Could you check a few things on this model? Use its own coordinates, in mm. A direction names the side the tool comes from. Round coordinates to 2 decimals unless told otherwise and drop trailing zeros. Loops run counter-clockwise (first coordinate to the right, second up) from the corner with the lowest first, then second, coordinate; pieces in that order, holes last.
from build123d import *

# Parameters (mm, degrees)
SKETCH1_R           = 18.875
SKETCH1_R_2         = 15.875
BOSS_EXTRUDE1_DEPTH = 47.85
SKETCH2_R           = 38
BOSS_EXTRUDE2_DEPTH = 30
SKETCH3_R           = 15.875
CUT_EXTRUDE1_DEPTH  = 47.85
SKETCH4_W           = 76
SKETCH4_H           = 20
CUT_EXTRUDE2_DEPTH  = 47.85
SKETCH5_R           = 2.65
CUT_EXTRUDE3_DEPTH  = 47.85
SKETCH11_R          = 1
CUT_EXTRUDE4_DEPTH  = 30
SKETCH12_R          = 4.7625
CUT_EXTRUDE5_DEPTH  = 8
SKETCH13_W          = 2.1
SKETCH13_H          = 3.2
SKETCH13_W_2        = 4.5
SKETCH13_H_2        = 2.2
SKETCH18_R          = 3.125
CUT_EXTRUDE8_DEPTH  = 30
SKETCH19_R          = 5.25
CUT_EXTRUDE9_DEPTH  = 27
SKETCH27_R          = 6.225
CUT_EXTRUDE12_DEPTH = 1.6
CHAMFER1_SIZE       = 2
SKETCH28_W          = 76
SKETCH28_H          = 20
CUT_EXTRUDE13_DEPTH = 1


with BuildPart() as part:
    # Sketch1 → Boss-Extrude1 (new body)
    with BuildSketch(Plane.XY):
        Circle(SKETCH1_R)
        Circle(SKETCH1_R_2, mode=Mode.SUBTRACT)
    extrude(amount=BOSS_EXTRUDE1_DEPTH)

    # Sketch2 → Boss-Extrude2 (add)
    with BuildSketch(Plane.XY.offset(47.85)):
        Circle(SKETCH2_R)
    extrude(amount=BOSS_EXTRUDE2_DEPTH)

    # Sketch3 → Cut-Extrude1 (cut)
    with BuildSketch(Plane(origin=(0, 0, 47.85), x_dir=(-1, 0, 0), z_dir=(0, 0, -1))):
        with Locations(Location((0, 0, 0), (0, 0, 180))):
            Circle(SKETCH3_R)
    extrude(amount=-CUT_EXTRUDE1_DEPTH, mode=Mode.SUBTRACT)

    # Sketch4 → Cut-Extrude2 (cut)
    with BuildSketch(Plane(origin=(0, 0, 0), x_dir=(1, 0, 0), z_dir=(0, 1, 0))):
        with Locations((0, -67.85)):
            Rectangle(SKETCH4_W, SKETCH4_H)
    extrude(amount=-CUT_EXTRUDE2_DEPTH, mode=Mode.SUBTRACT)

    # Sketch5 → Cut-Extrude3 (cut)
    with BuildSketch(Plane(origin=(0, 0, 0), x_dir=(-1, 0, 0), z_dir=(0, -1, 0))):
        with Locations(Location((26.9375, -67.85, 0), (0, 0, 90))):
            Circle(SKETCH5_R)
        with Locations(Location((-26.9375, -67.85, 0), (0, 0, 90))):
            Circle(SKETCH5_R)
    extrude(amount=-CUT_EXTRUDE3_DEPTH, mode=Mode.SUBTRACT)

    # Sketch11 → Cut-Extrude4 (cut)
    with BuildSketch(Plane.XY.offset(77.85)):
        with Locations((0, 28.5)):
            Circle(SKETCH11_R)
    extrude(amount=-CUT_EXTRUDE4_DEPTH, mode=Mode.SUBTRACT)

    # Sketch12 → Cut-Extrude5 (cut)
    with BuildSketch(Plane.XY.offset(77.85)):
        with Locations((0, 28.5)):
            Circle(SKETCH12_R)
    extrude(amount=-CUT_EXTRUDE5_DEPTH, mode=Mode.SUBTRACT)

    # Sketch13 → Cut-Revolve1 (revolve, cut)
    with BuildSketch(Plane(origin=(0, 0, 0), x_dir=(0, 0, -1), z_dir=(1, 0, 0)), mode=Mode.PRIVATE) as cut_revolve1_sk:
        with Locations((-14.85, 18.875)):
            Rectangle(SKETCH13_W, SKETCH13_H)
        with Locations((-22.85, 18.875)):
            Rectangle(SKETCH13_W, SKETCH13_H)
        with Locations((-35.85, 18.875)):
            Rectangle(SKETCH13_W, SKETCH13_H)
        with Locations((-39.85, 18.875)):
            Rectangle(SKETCH13_W, SKETCH13_H)
        with Locations((-29.85, 18.375)):
            Rectangle(SKETCH13_W_2, SKETCH13_H_2)
    revolve(cut_revolve1_sk.sketch.rotate(Axis((0, 0, 0), (0, 0, 1)), 90), axis=Axis((0, 0, 0), (0, 0, 1)), mode=Mode.SUBTRACT)

    # Sketch18 → Cut-Extrude8 (cut)
    with BuildSketch(Plane.XY.offset(77.85)):
        with Locations((27.105110714, 8.80698434)):
            Circle(SKETCH18_R)
        with Locations((16.75187969, -23.05698434)):
            Circle(SKETCH18_R)
        with Locations((-16.75187969, -23.05698434)):
            Circle(SKETCH18_R)
        with Locations((-27.105110714, 8.80698434)):
            Circle(SKETCH18_R)
    extrude(amount=-CUT_EXTRUDE8_DEPTH, mode=Mode.SUBTRACT)

    # Sketch19 → Cut-Extrude9 (cut)
    with BuildSketch(Plane.XY.offset(77.85)):
        with Locations((27.105110714, 8.80698434)):
            Circle(SKETCH19_R)
        with Locations((16.75187969, -23.05698434)):
            Circle(SKETCH19_R)
        with Locations((-16.75187969, -23.05698434)):
            Circle(SKETCH19_R)
        with Locations((-27.105110714, 8.80698434)):
            Circle(SKETCH19_R)
    extrude(amount=-CUT_EXTRUDE9_DEPTH, mode=Mode.SUBTRACT)

    # Sketch27 → Cut-Extrude12 (cut)
    with BuildSketch(Plane(origin=(0, 0, 47.85), x_dir=(-1, 0, 0), z_dir=(0, 0, -1))):
        with Locations((0, 28.5)):
            Circle(SKETCH27_R)
    extrude(amount=-CUT_EXTRUDE12_DEPTH, mode=Mode.SUBTRACT)

    # Chamfer1
    chamfer1_edges = [part.edges().sort_by_distance(p)[0] for p in [
        (0, 38, 77.85),
    ]]
    chamfer(chamfer1_edges, length=CHAMFER1_SIZE)

    # Sketch28 → Cut-Extrude13 (cut)
    with BuildSketch(Plane(origin=(0, 0, 0), x_dir=(-1, 0, 0), z_dir=(0, -1, 0))):
        with Locations((0, -67.85)):
            Rectangle(SKETCH28_W, SKETCH28_H)
    extrude(amount=-CUT_EXTRUDE13_DEPTH, mode=Mode.SUBTRACT)


solid = part.part
Item 1: For faces 1 (the flat face through (-17.4, -7.9, 47.85)), 2 (the flat face through (-29, 1, 65)), 3 (the flat face through (17, 6, 13.8)), 4 (the cylindrical face through (-0.13, 29.49, 59.79)), which set-ups out of +Z, -Z, +X, -X, +Y, -Y let a thin tool reach every point of the face, with its end or its side?
Results list:
face 1: -Z
face 2: +Z, +X, -X, -Y
face 3: none
face 4: +Z, -Z
Item 2: We'd pull the mould along Y, two halves only. Please class faces 5 (the cylindrical face through (-29.59, 6.91, 49.37)), 6 (the cylindrical face through (12.88, -19.51, 54.4)), 7 (the cylindrical face through (18.003, 5.67, 18.809)), 8 (the flat face through (17, 6, 36.9)): released by +Y, released by -Y, zero draft, split by the parting line, or undercut.
Results list:
face 5: undercut
face 6: undercut
face 7: split by the parting line
face 8: zero draft
Item 3: If we section it at C-C, the plane z = 54.5: Please give me the cut outline in (x, y) (3 decimals).
Results list:
outline: circle Ø76 at (0, 0); hole circle Ø10.5 at (-27.105, 8.807); hole circle Ø10.5 at (-16.752, -23.057); hole circle Ø31.75 at (0, 0); hole circle Ø2 at (0, 28.5); hole circle Ø10.5 at (16.752, -23.057); hole circle Ø10.5 at (27.105, 8.807)
Item 4: If I drill on line 1 along X through (y, z) = (21, 70); line 2 along Y through (x, z) = (0, 62) (3 decimals); line 3 along Y through (x, z) = (0, 72.5) (1 decimal), over which ranges is the centre line in solid material (lowest first)?
Results list:
line 1: x = -31.67 to -28.49, -25.39 to 25.39, 28.49 to 31.67
line 2: y = 15.875 to 27.5, 29.5 to 38
line 3: y = 15.9 to 23.7, 33.3 to 38
Item 5: Will these pins go through, and if not, where does the flat tip stop? pin 1 (16 mm diameter, centred on x = -31.5, z = 71, fed in from -Y); pin 2 (5 mm diameter, centred on y = -13.5, z = 38, fed in from +X); pin 3 (17 mm diameter, centred on x = -27.11, y = 8.81, fed in from -Z).
Results list:
pin 1: stops at y = 1
pin 2: stops at x = 15.34
pin 3: stops at z = 47.85
Item 6: If we section it at B-B, the plane z = 11: Please give me the cut outline in (x, y) (3 decimals), then the cut area to 3 significant figures.
Results list:
outline: circle Ø37.75 at (0, 0); hole circle Ø31.75 at (0, 0)
area: 328 mm2
Item 7: If we section it at A-A, the plane z = 67.85: Count the separate pieces of the cut face and the enclosed holes in it, then the cut area to 3 significant figures.
Results list:
separate pieces: 3
enclosed holes: 1
area: 1,490 mm2
